The figure shows three views and two pictorial views of one solid part (mm, origin at its lowest corner). Answer the questions. Round coordinates to 2 decimals unless told otherwise and drop trailing zeros. Write each loop counter-clockwise with the first axis right and the second up, starting at its lowest first coordinate (ties: lowest second). Pieces come first, ordered by that corner, then holes. Notation, with made-up numbers: M 5.25,-14.75 L 43.25,-14.75 A21 ccw 43.25,-6.75 Z; hole C 34.25,25.5 d4. An arc over 180 degrees is marked long. Answer in a Markdown table with one row per item.
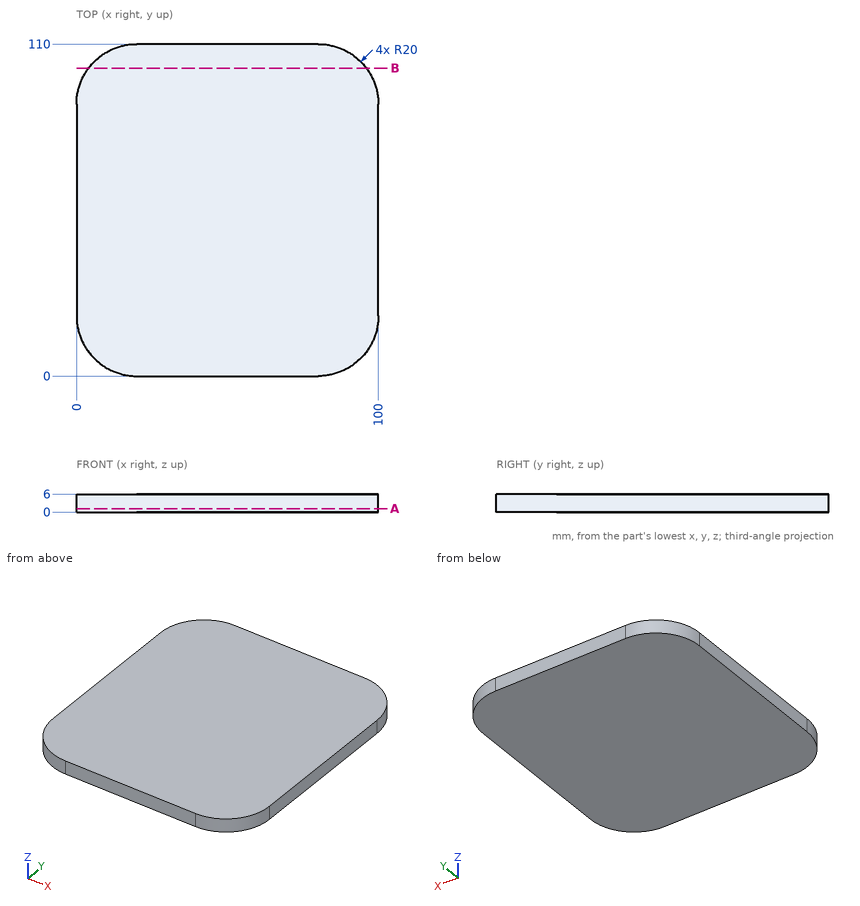
1. Consider line 1 along Y through (x, z) = (90, 1.5); line 2 along X through (y, z) = (18, 1.9); line 3 along Y through (x, z) = (6, 2.45). Determine where each line is inside the solid, lowest interval first. Write a range as from..to.
Calculated:
| item | result |
|---|---|
| line 1 | y = 2.68..107.32 |
| line 2 | x = 0.1..99.9 |
| line 3 | y = 5.72..104.28 |
2. The part is cut by section A-A (z = 1.15). Determine the outline of the cut face in (x, y), plus the area to 3 significant figures.
Calculated:
| item | result |
|---|---|
| outline | M 0,20 A20 ccw 20,0 L 80,0 A20 ccw 100,20 L 100,90 A20 ccw 80,110 L 20,110 A20 ccw 0,90 Z |
| area | 10,700 mm² |
3. The part is cut by section B-B (y = 102). Determine the outline of the cut face in (x, z), plus the area to 3 significant figures.
Calculated:
| item | result |
|---|---|
| outline | M 4,0 L 96,0 L 96,6 L 4,6 Z |
| area | 552 mm² |
4. Given pin 1 (2 mm diameter, centred on y = 68, z = 3, fed in from -X), flat-ended and moving along its own axis, determine where the tip first touches the part or whether it passes through.
Calculated:
| item | result |
|---|---|
| pin 1 | stops at x = 0 |
